Autodesk Inventor part; units mm, degrees
ref_plane "YZ Plane" through (0, 0, 0) normal (1, 0, 0) x (0, 1, 0)
ref_plane "XZ Plane" through (0, 0, 0) normal (0, 1, 0) x (-1, 0, 0)
ref_plane "XY Plane" through (0, 0, 0) normal (0, 0, 1) x (1, 0, 0)
sketch "Sketch2" plane through (0, 0, 0) normal (0, 0, 1) x (1, 0, 0)
  circle A0 centre (0, 0) radius 45
  dimension "d0" = 90
extrude "Extrusion1" add sketch "Sketch2" along normal blind 10
sketch "Sketch4" plane through (0, 0, 10) normal (0, 0, 1) x (1, 0, 0)
  circle A0 centre (0, 0) radius 11.5
  dimension "d14" = 23
extrude "Extrusion3" add sketch "Sketch4" along normal blind 23
sketch "Sketch5" plane through (0, 0, 33) normal (0, 0, 1) x (1, 0, 0)
  circle A0 centre (-8, 0) radius 2
  circle A1 centre (0, 0) radius 3.5
  circle A2 centre (0, 0) radius 11.5 construction
  circle A3 centre (-2.4721, -7.6085) radius 2
  circle A4 centre (6.4721, -4.7023) radius 2
  circle A5 centre (6.4721, 4.7023) radius 2
  circle A6 centre (-2.4721, 7.6085) radius 2
  dimension "d19" = 4
  dimension "d20" = 8
  dimension "d21" = 360
  dimension "d22" = 7
extrude "Extrusion4" cut sketch "Sketch5" against normal through all
sketch "Sketch6" plane through (0, 0, 10) normal (0, 0, 1) x (1, 0, 0)
  line L0 (-40, 0) -> (-27.3, 0)
  line L1 (-27.3, 0) -> (-27.3, 12.7)
  line L2 (-27.3, 12.7) -> (-40, 12.7)
  line L3 (-40, 12.7) -> (-40, 0)
  line L4 (-40.5, 13.2) -> (-26.8, 13.2)
  line L5 (-26.8, 13.2) -> (-26.8, -0.5)
  line L6 (-26.8, -0.5) -> (-40.5, -0.5)
  line L7 (-40.5, -0.5) -> (-40.5, 13.2)
  line L8 (-33.6501, -21.6256) -> (-22.9662, -14.7595)
  line L9 (-22.9662, -14.7595) -> (-29.8324, -4.0756)
  line L10 (-29.8324, -4.0756) -> (-40.5163, -10.9417)
  line L11 (-40.5163, -10.9417) -> (-33.6501, -21.6256)
  line L12 (-41.2072, -10.7914) -> (-29.6821, -3.3846)
  line L13 (-29.6821, -3.3846) -> (-22.2753, -14.9098)
  line L14 (-22.2753, -14.9098) -> (-33.8004, -22.3166)
  line L15 (-33.8004, -22.3166) -> (-41.2072, -10.7914)
  line L16 (-16.6166, -36.3853) -> (-11.3408, -24.833)
  line L17 (-11.3408, -24.833) -> (-22.8932, -19.5572)
  line L18 (-22.8932, -19.5572) -> (-28.1689, -31.1095)
  line L19 (-28.1689, -31.1095) -> (-16.6166, -36.3853)
  line L20 (-28.8315, -31.3566) -> (-23.1403, -18.8947)
  line L21 (-23.1403, -18.8947) -> (-10.6783, -24.5858)
  line L22 (-10.6783, -24.5858) -> (-16.3695, -37.0478)
  line L23 (-16.3695, -37.0478) -> (-28.8315, -31.3566)
  line L24 (5.6926, -39.5929) -> (3.8852, -27.0221)
  line L25 (3.8852, -27.0221) -> (-8.6855, -28.8295)
  line L26 (-8.6855, -28.8295) -> (-6.8781, -41.4003)
  line L27 (-6.8781, -41.4003) -> (5.6926, -39.5929)
  line L28 (-7.3019, -41.9663) -> (-9.2516, -28.4058)
  line L29 (-9.2516, -28.4058) -> (4.3089, -26.4561)
  line L30 (4.3089, -26.4561) -> (6.2587, -40.0166)
  line L31 (6.2587, -40.0166) -> (-7.3019, -41.9663)
  line L32 (26.1944, -30.23) -> (17.8777, -20.632)
  line L33 (17.8777, -20.632) -> (8.2797, -28.9487)
  line L34 (8.2797, -28.9487) -> (16.5964, -38.5467)
  line L35 (16.5964, -38.5467) -> (26.1944, -30.23)
  line L36 (16.546, -39.252) -> (7.5744, -28.8983)
  line L37 (7.5744, -28.8983) -> (17.9281, -19.9267)
  line L38 (17.9281, -19.9267) -> (26.8997, -30.2804)
  line L39 (26.8997, -30.2804) -> (16.546, -39.252)
  line L40 (38.3797, -11.2693) -> (26.1942, -7.6913)
  line L41 (26.1942, -7.6913) -> (22.6162, -19.8769)
  line L42 (22.6162, -19.8769) -> (34.8017, -23.4549)
  line L43 (34.8017, -23.4549) -> (38.3797, -11.2693)
  line L44 (35.1406, -24.0755) -> (21.9955, -20.2157)
  line L45 (21.9955, -20.2157) -> (25.8553, -7.0707)
  line L46 (25.8553, -7.0707) -> (39.0003, -10.9304)
  line L47 (39.0003, -10.9304) -> (35.1406, -24.0755)
  line L48 (38.3797, 11.2693) -> (26.1942, 7.6913)
  line L49 (26.1942, 7.6913) -> (29.7722, -4.4943)
  line L50 (29.7722, -4.4943) -> (41.9577, -0.9163)
  line L51 (41.9577, -0.9163) -> (38.3797, 11.2693)
  line L52 (42.5783, -1.2551) -> (29.4333, -5.1149)
  line L53 (29.4333, -5.1149) -> (25.5735, 8.0302)
  line L54 (25.5735, 8.0302) -> (38.7186, 11.8899)
  line L55 (38.7186, 11.8899) -> (42.5783, -1.2551)
  line L56 (26.1944, 30.23) -> (17.8777, 20.632)
  line L57 (17.8777, 20.632) -> (27.4757, 12.3152)
  line L58 (27.4757, 12.3152) -> (35.7924, 21.9133)
  line L59 (35.7924, 21.9133) -> (26.1944, 30.23)
  line L60 (36.4978, 21.9637) -> (27.5262, 11.6099)
  line L61 (27.5262, 11.6099) -> (17.1724, 20.5815)
  line L62 (17.1724, 20.5815) -> (26.144, 30.9353)
  line L63 (26.144, 30.9353) -> (36.4978, 21.9637)
  line L64 (5.6926, 39.5929) -> (3.8852, 27.0221)
  line L65 (3.8852, 27.0221) -> (16.4559, 25.2147)
  line L66 (16.4559, 25.2147) -> (18.2633, 37.7855)
  line L67 (18.2633, 37.7855) -> (5.6926, 39.5929)
  line L68 (18.8294, 38.2092) -> (16.8797, 24.6487)
  line L69 (16.8797, 24.6487) -> (3.3191, 26.5984)
  line L70 (3.3191, 26.5984) -> (5.2688, 40.1589)
  line L71 (5.2688, 40.1589) -> (18.8294, 38.2092)
  line L72 (-16.6166, 36.3853) -> (-11.3408, 24.833)
  line L73 (-11.3408, 24.833) -> (0.2115, 30.1087)
  line L74 (0.2115, 30.1087) -> (-5.0643, 41.6611)
  line L75 (-5.0643, 41.6611) -> (-16.6166, 36.3853)
  line L76 (-4.8172, 42.3236) -> (0.874, 29.8616)
  line L77 (0.874, 29.8616) -> (-11.5879, 24.1704)
  line L78 (-11.5879, 24.1704) -> (-17.2791, 36.6324)
  line L79 (-17.2791, 36.6324) -> (-4.8172, 42.3236)
  line L80 (-33.6501, 21.6256) -> (-22.9662, 14.7595)
  line L81 (-22.9662, 14.7595) -> (-16.1001, 25.4434)
  line L82 (-16.1001, 25.4434) -> (-26.784, 32.3096)
  line L83 (-26.784, 32.3096) -> (-33.6501, 21.6256)
  line L84 (-26.9343, 33.0005) -> (-15.4091, 25.5937)
  line L85 (-15.4091, 25.5937) -> (-22.8159, 14.0685)
  line L86 (-22.8159, 14.0685) -> (-34.3411, 21.4753)
  line L87 (-34.3411, 21.4753) -> (-26.9343, 33.0005)
  point P0 (0, 0)
  dimension "d25" = 12.7
  dimension "d26" = 12.7
  dimension "d27" = 40
  dimension "d28" = 0.5
  dimension "d31" = 360
extrude "Extrusion5" cut sketch "Sketch6" against normal blind 6.35 contours L3 L2 L1 L0 | L4 L5 L6 L7 | L11 L10 L9 L8 | L12 L13 L14 L15 | L19 L18 L17 L16 | L20 L21 L22 L23 | L27 L26 L25 L24 | L28 L29 L30 L31 | L35 L34 L33 L32 | L36 L37 L38 L39 | L43 L42 L41 L40 | L44 L45 L46 L47 | L51 L50 L49 L48 | L52 L53 L54 L55 | L59 L58 L57 L56 | L60 L61 L62 L63 | L67 L66 L65 L64 | L68 L69 L70 L71 | L75 L74 L73 L72 | L76 L77 L78 L79 | L83 L82 L81 L80 | L84 L85 L86 L87
properties part number "SG02" material "ABS Plastic"
CAD build for the part. Positions are in the model's coordinates, mm. A direction names the side the tool comes from. Coordinates: 2 decimals unless noted, no trailing zeros. Loops run counter-clockwise (first coordinate to the right, second up) from the corner with the lowest first, then second, coordinate; pieces in that order, holes last. Notation, with made-up numbers: (13.5, 16.5) - (31.5, 16.5) arc R26 cw to (31.5, 40.5) - close; hole circle Ø1 at (38, -33). An arc over 180 degrees is marked (long way). Return JSON: item names as keys, results as strings.
1. Band-saw the part on A-A (x = -38). Give the cut face in (y, z).
Result:
{"outline": "(-24.1, 0) - (24.1, 0) - (24.1, 10) - (13.2, 10) - (13.2, 3.65) - (-0.5, 3.65) - (-0.5, 10) - (-8.73, 10) - (-8.73, 3.65) - (-15.78, 3.65) - (-15.78, 10) - (-24.1, 10) - close"}
2. 3-axis set-ups, long thin cutter, end or side, ignore diameter. For faces 1 (the cylindrical face through (-4.47, 7.7, 16.73)), 2 (the flat face through (17, -29, 3.65)): which of +Z, -Z, +X, -X, +Y, -Y reach the whole face in a straight line?
Result:
{"face 1": "+Z, -Z", "face 2": "+Z"}
3. Band-saw the part on C-C (z = 8). State how many separate pieces and enclosed holes the cut face has, and give its area (3 significant figures).
Result:
{"separate pieces": "1", "enclosed holes": "17", "area": "4,200 mm2"}
4. Drop flat-ended pins along their axis: pin 1 (12 mm diameter, centred on x = -25.5, z = 10.5, fed in from -Y); pin 2 (4 mm diameter, centred on y = -4.5, z = 27.5, fed in from +X) (3 decimals); pin 3 (3 mm diameter, centred on x = -2.47, y = 7.61, fed in from +Z); pin 4 (3 mm diameter, centred on y = 7.5, z = 7, fed in from -X). Give the stop position or say it passes through.
Result:
{"pin 1": "stops at y = -40.55", "pin 2": "stops at x = 11.225", "pin 3": "passes through", "pin 4": "stops at x = -44.6"}
5. Band-saw the part on B-B (z = 27). Give the cut face in (x, y), and give its area (3 significant figures).
Result:
{"outline": "circle Ø23 at (0, 0); hole circle Ø4 at (-8, 0); hole circle Ø4 at (-2.47, -7.61); hole circle Ø4 at (-2.47, 7.61); hole circle Ø7 at (0, 0); hole circle Ø4 at (6.47, -4.7); hole circle Ø4 at (6.47, 4.7)", "area": "314 mm2"}
6. Probe L1, parallel to Y at x = -13, z = 8; L2, parallel to X at y = -6.5, z = 3.5; L3, parallel to Y at x = 0, z = 12. List the from-to ranges inside material, lowest first. Write a range as from..to.
Result:
{"L1": "y = -43.08..-29.67, -23.53..27.26, 38.59..43.08", "L2": "x = -44.53..-4.14, -0.81..5.6, 7.35..44.53", "L3": "y = -11.5..-3.5, 3.5..11.5"}
